```python
from build123d import *

# Parameters (mm, degrees)
ESBO_O1_W                  = 151
ESBO_O1_H                  = 62
RESSALTO_EXTRUS_O1_DEPTH   = 35.6
ESBO_O2_W                  = 145
ESBO_O2_H                  = 56
CORTE_EXTRUS_O1_DEPTH      = 33.1
ESBO_O3_W                  = 122
ESBO_O3_H                  = 62
CORTE_EXTRUS_O2_DEPTH      = 13.1
CHANFRO1_SIZE              = 5
ESBO_O7_R                  = 0.7
CORTE_EXTRUS_O6_DEPTH      = 3
ESBO_O6_R                  = 0.75
RESSALTO_EXTRUS_O2_DEPTH   = 35.6
FILETE1_R                  = 3
CHANFRO2_SIZE              = 1
ESBO_O8_W                  = 5
ESBO_O8_H                  = 3
RESSALTO_EXTRUS_O3_DEPTH   = 3
CORTE_EXTRUS_O7_DEPTH      = 3
CORTE_EXTRUS_O7_DEPTH_BACK = 5
ESBO_O9_W                  = 13
ESBO_O9_H                  = 22


with BuildPart() as part:
    # Esboço1 → Ressalto-extrusão1 (new body)
    with BuildSketch(Plane(origin=(0, 0, 0), x_dir=(1, 0, 0), z_dir=(0, 1, 0))):
        with Locations((75.5, 31)):
            Rectangle(ESBO_O1_W, ESBO_O1_H)
    extrude(amount=RESSALTO_EXTRUS_O1_DEPTH)

    # Esboço2 → Corte-extrusão1 (cut)
    with BuildSketch(Plane(origin=(0, 35.6, 0), x_dir=(1, 0, 0), z_dir=(0, 1, 0))):
        with Locations((75.5, 31)):
            Rectangle(ESBO_O2_W, ESBO_O2_H)
    extrude(amount=-CORTE_EXTRUS_O1_DEPTH, mode=Mode.SUBTRACT)

    # Esboço3 → Corte-extrusão2 (cut)
    with BuildSketch(Plane(origin=(0, 35.6, 0), x_dir=(1, 0, 0), z_dir=(0, 1, 0))):
        with Locations((61, 31)):
            Rectangle(ESBO_O3_W, ESBO_O3_H)
    extrude(amount=-CORTE_EXTRUS_O2_DEPTH, mode=Mode.SUBTRACT)

    # Chanfro1
    # the kernel refuses this chamfer: 5 mm, written as the material it takes off along each edge
    with BuildSketch(Plane(origin=(0, 22.5, -74.85841494), x_dir=(0.9996219169112968, 0.027495876610586317, 0), z_dir=(0, 0, 1))) as chanfro1_piece_1:
        Polygon((CHANFRO1_SIZE * 0.999621916911, -CHANFRO1_SIZE * 0.0274958766106), (-CHANFRO1_SIZE * 0.0274958766106, -CHANFRO1_SIZE * 0.999621916911), (0, 0), align=None)
    extrude(amount=87.71682988, mode=Mode.SUBTRACT)

    # Esboço7 → Corte-extrusão6 (cut)
    with BuildSketch(Plane(origin=(151, 0, 0), x_dir=(0, 0, -1), z_dir=(1, 0, 0))):
        with Locations((31, 29.6)):
            Circle(ESBO_O7_R)
    extrude(amount=-CORTE_EXTRUS_O6_DEPTH, mode=Mode.SUBTRACT)

    # Esboço6 → Ressalto-extrusão2 (add)
    with BuildSketch(Plane(origin=(0, 35.6, 0), x_dir=(1, 0, 0), z_dir=(0, 1, 0))):
        with Locations((146, 62)):
            Circle(ESBO_O6_R)
        with Locations((146, 0)):
            Circle(ESBO_O6_R)
    extrude(amount=-RESSALTO_EXTRUS_O2_DEPTH)

    # Filete1
    filete1_edges = [part.edges().sort_by_distance(p)[0] for p in [
        (122, 35.6, -60.5),
        (122, 35.6, -1.5),
    ]]
    fillet(filete1_edges, radius=FILETE1_R)

    # Chanfro2
    chanfro2_edges = [part.edges().sort_by_distance(p)[0] for p in [
        (0, 8.75, 0),
        (0, 8.75, -62),
        (0, 0, -31),
    ]]
    chamfer(chanfro2_edges, length=CHANFRO2_SIZE)

    # Esboço8 → Ressalto-extrusão3 (add)
    with BuildSketch(Plane(origin=(0, 22.5, 0), x_dir=(1, 0, 0), z_dir=(0, 1, 0))):
        with Locations((12.5, 60.5)):
            Rectangle(ESBO_O8_W, ESBO_O8_H)
        with Locations((12.5, 1.5)):
            Rectangle(ESBO_O8_W, ESBO_O8_H)
        with Locations((109.5, 60.5)):
            Rectangle(ESBO_O8_W, ESBO_O8_H)
        with Locations((109.5, 1.5)):
            Rectangle(ESBO_O8_W, ESBO_O8_H)
    extrude(amount=RESSALTO_EXTRUS_O3_DEPTH)

    # Esboço9 → Corte-extrusão7 (cut, two sides: drawn at the far end of the back side and taken through both)
    with BuildSketch(Plane(origin=(0, 22.5, 0), x_dir=(1, 0, 0), z_dir=(0, 1, 0)).offset(-CORTE_EXTRUS_O7_DEPTH_BACK)):
        with Locations((6.5, 49)):
            Rectangle(ESBO_O9_W, ESBO_O9_H)
    extrude(amount=CORTE_EXTRUS_O7_DEPTH + CORTE_EXTRUS_O7_DEPTH_BACK, mode=Mode.SUBTRACT)


solid = part.part
```
Geometry: final body of the model. Coordinates: model frame, mm. A direction names the side the tool comes from. Give positions to 0.01 mm unless a question says otherwise; leave off trailing zeros. Loops run counter-clockwise (first coordinate to the right, second up) from the corner with the lowest first, then second, coordinate; pieces in that order, holes last. Notation, with made-up numbers: (-9, -18) - (-4, -18) arc R26 cw to (-4, 2) - close; hole circle Ø9 at (74, 1). An arc over 180 degrees is marked (long way). Answer as CSV lines item,"result". Start each with the question number.
(1) Section query B-B (x = 130.5). Output: boundary loops of the cut face in (y, z), and give its area (3 significant figures).
(2) Pin query (flat end, axial travel): P1, Ø2.5, axis at x = 11.5, z = -60.5, coming from the +Y side; P2, Ø6, axis at x = 34, y = 8, coming from the -Z side; P3, Ø2.5, axis at x = 118, z = -1, coming from the +Y side. Return the tip coordinate at first contact, or that it passes through.
(3) Section query A-A (y = 5). Output: boundary loops of the cut face in (x, z).
(4) Mould query, pull axis Z, two halves, no side actions, for faces 6 (the face through (12, 25.5, -2)), 7 (the face through (3, 12, -31)), 8 (the face through (72, 14, -62)). Classes: +Z half, -Z half, draft (parallel to the pull), parting line (faces both ways), or undercut.
(5) Section query D-D (y = 27). Output: boundary loops of the cut face in (x, z), and give its area (3 significant figures).
(6) Section query C-C (z = -42). Output: boundary loops of the cut face in (x, y), and give its area (3 significant figures).
(7) Ray query, line 1 along Z through (x, y) = (24, 8); line 2 along X through (y, z) = (13, -54); line 3 along Y through (x, z) = (149.85, -31). Return the intervals inside material, ascending. Write a range as [from, to].
(8) Reachability of faces 1 (the face through (74, 16, -3)), 2 (the face through (109, 25.5, -61)), 3 (the face through (15, 24, -1)), 4 (the face through (149, 18, -62)), 5 (the face through (149, 35.6, -34)) from +Z, -Z, +X, -X, +Y, -Y: full face, straight path, thin tool, end or side. Return the list, or none.
Worked answers:
1,outline,"(0, -62) - (35.6, -62) - (35.6, -59) - (2.5, -59) - (2.5, -3) - (35.6, -3) - (35.6, 0) - (0, 0) - close"
1,area,"354 mm^2"
2,P1,"stops at y = 25.5"
2,P2,"stops at z = -62"
2,P3,"stops at y = 22.5"
3,outline,"(0, -61) - (1, -62) - (145.25, -62) arc R0.75 ccw to (146.75, -62) - (151, -62) - (151, 0) - (146.75, 0) arc R0.75 ccw to (145.25, 0) - (1, 0) - (0, -1) - close; hole (3, -59) - (148, -59) - (148, -3) - (3, -3) - close"
4,face 6,"draft"
4,face 7,"undercut"
4,face 8,"-Z half"
5,outline,"(122, -62) - (145.25, -62) arc R0.75 ccw to (146.75, -62) - (151, -62) - (151, 0) - (146.75, 0) arc R0.75 ccw to (145.25, 0) - (122, 0) - (122, -3) - (148, -3) - (148, -59) - (122, -59) - close"
5,area,"344 mm^2"
6,outline,"(0, 1) - (1, 0) - (151, 0) - (151, 35.6) - (148, 35.6) - (148, 2.5) - (3, 2.5) - (3, 17.5) - (0, 17.5) - close"
6,area,"521 mm^2"
7,line 1,"z = [-62, -59], [-3, 0]"
7,line 2,"x = [0, 3], [148, 151]"
7,line 3,"y = [0, 28.9], [30.3, 35.6]"
8,face 1,"+Y"
8,face 2,"+Z, -Z, -X, +Y"
8,face 3,"+Z, -Z, +Y"
8,face 4,"-Z, +X, +Y, -Y"
8,face 5,"+Z, -Z, +X, -X, +Y"
